Verification items for the finished model (mm, model axes). A direction names the side the tool comes from. Coordinates: 2 decimals unless noted, no trailing zeros. Write each loop counter-clockwise with the first axis right and the second up, starting at its lowest first coordinate (ties: lowest second). Pieces come first, ordered by that corner, then holes. Notation, with made-up numbers: (69.25, 61) -> (74.25, 61) arc R32 cw to (74.25, 95) -> close; hole circle Ø6 at (-19, 20). An arc over 180 degrees is marked (long way). Answer in a Markdown table with one row per item.
```python
from build123d import *

# Parameters (mm, degrees)
SKETCH038_W      = 110
SKETCH038_H      = 32.6
PAD020_DEPTH     = 5
SKETCH039_R      = 1.6
POCKET018_DEPTH  = 5
SKETCH040_W      = 10
SKETCH040_H      = 21.4
SKETCH040_H_2    = 10
PAD021_DEPTH     = 35
MIRROREDSKETCH_R = 1.6
PAD022_DEPTH     = 5
POCKET019_DEPTH  = 110
FILLET012_R      = 2.5


with BuildPart() as part:
    # Sketch038 → Pad020 (new body)
    with BuildSketch(Plane.XY):
        Rectangle(SKETCH038_W, SKETCH038_H)
    extrude(amount=-PAD020_DEPTH)

    # Sketch039 (on Face6 of Pad020) → Pocket018 (cut)
    with BuildSketch(Plane(origin=(0, 0, -5), x_dir=(1, 0, 0), z_dir=(0, 0, -1))):
        with Locations((-37.5, 11.5)):
            Circle(SKETCH039_R)
        with Locations((-37.5, -11.5)):
            Circle(SKETCH039_R)
        with Locations((37.5, -11.5)):
            Circle(SKETCH039_R)
        with Locations((37.5, 11.5)):
            Circle(SKETCH039_R)
    extrude(amount=-POCKET018_DEPTH, mode=Mode.SUBTRACT)

    # Sketch040 (on Face4 of Pocket018) → Pad021 (join)
    with BuildSketch(Plane.XY):
        with Locations((-50, 17)):
            Rectangle(SKETCH040_W, SKETCH040_H)
        with Locations((50, 17)):
            Rectangle(SKETCH040_W, SKETCH040_H)
        with Locations((50, -11.3)):
            Rectangle(SKETCH040_W, SKETCH040_H_2)
        with Locations((-50, -11.3)):
            Rectangle(SKETCH040_W, SKETCH040_H_2)
    extrude(amount=-PAD021_DEPTH)

    # MirroredSketch (on Face35 of Pad021) → Pad022 (join)
    with BuildSketch(Plane(origin=(0, 0, -35), x_dir=(1, 0, 0), z_dir=(0, 0, -1))):
        with BuildLine():
            Line((-45, -27.7), (-45, -6.3))
            Line((-45, -6.3), (-55, -6.3))
            Line((-55, -6.3), (-55, -27.7))
            Line((-55, -27.7), (-55, -30.7))
            ThreePointArc((-55, -30.7), (-50, -35.7), (-45, -30.7))
            Line((-45, -27.7), (-45, -30.7))
        make_face()
        with Locations((-50, -30.7)):
            Circle(MIRROREDSKETCH_R, mode=Mode.SUBTRACT)
        with BuildLine():
            Line((55, -27.7), (55, -6.3))
            Line((55, -6.3), (45, -6.3))
            Line((45, -6.3), (45, -27.7))
            Line((45, -27.7), (45, -30.7))
            ThreePointArc((45, -30.7), (49.999989, -35.7), (55, -30.700021))
            Line((55, -27.7), (55, -30.700021))
        make_face()
        with Locations((50, -30.7)):
            Circle(MIRROREDSKETCH_R, mode=Mode.SUBTRACT)
        with BuildLine():
            Line((45, 6.3), (55, 6.3))
            Line((55, 6.3), (55, 16.3))
            Line((55, 16.3), (55, 19.3))
            ThreePointArc((55, 19.3), (50, 24.3), (45, 19.3))
            Line((45, 16.3), (45, 19.3))
            Line((45, 16.3), (45, 6.3))
        make_face()
        with Locations((50, 19.3)):
            Circle(MIRROREDSKETCH_R, mode=Mode.SUBTRACT)
        with BuildLine():
            Line((-55, 6.3), (-45, 6.3))
            Line((-45, 6.3), (-45, 16.3))
            Line((-45, 16.3), (-45, 19.3))
            ThreePointArc((-45, 19.3), (-50, 24.3), (-55, 19.3))
            Line((-55, 16.3), (-55, 19.3))
            Line((-55, 16.3), (-55, 6.3))
        make_face()
        with Locations((-50, 19.3)):
            Circle(MIRROREDSKETCH_R, mode=Mode.SUBTRACT)
    extrude(amount=PAD022_DEPTH)

    # Sketch041 (on Face44 of Pad022) → Pocket019 (cut)
    with BuildSketch(Plane.YZ.offset(55)):
        Polygon((16.3, 0), (27.7, -35), (27.7, 0), align=None)
        Polygon((17.7, -40), (6.3, -5), (6.3, -40), align=None)
    extrude(amount=-POCKET019_DEPTH, mode=Mode.SUBTRACT)

    # Fillet012
    fillet012_edges = [part.edges().sort_by_distance(p)[0] for p in [
        (-50, 6.3, -5),
        (50, 6.3, -5),
    ]]
    fillet(fillet012_edges, radius=FILLET012_R)


solid = part.part
```
1. Sectioned sample at A-A, the plane x = -50. Record the cut outline in (y, z), and give its area (3 significant figures).
Findings below:
| item | result |
|---|---|
| outline | (-24.3, -40) -> (-20.9, -40) -> (-20.9, -35) -> (-24.3, -35) -> close; (-17.7, -40) -> (-6.3, -40) -> (-6.3, -5) -> (4.49, -5) arc R2.5 cw to (6.86, -6.73) -> (17.7, -40) -> (29.1, -40) -> (29.1, -35) -> (27.7, -35) -> (16.3, 0) -> (-16.3, 0) -> (-16.3, -35) -> (-17.7, -35) -> close; (32.3, -40) -> (35.7, -40) -> (35.7, -35) -> (32.3, -35) -> close |
| area | 969 mm² |
2. Sectioned sample at C-C, the plane y = 20.5. Record the cut outline in (x, z).
Findings below:
| item | result |
|---|---|
| outline | (-55, -40) -> (-45, -40) -> (-45, -12.89) -> (-55, -12.89) -> close; (45, -40) -> (55, -40) -> (55, -12.89) -> (45, -12.89) -> close |
3. Sectioned sample at B-B, the plane z = -20. Record the cut outline in (x, y), and give its area (3 significant figures).
Findings below:
| item | result |
|---|---|
| outline | (-55, -16.3) -> (-45, -16.3) -> (-45, -6.3) -> (-55, -6.3) -> close; (-55, 11.19) -> (-45, 11.19) -> (-45, 22.81) -> (-55, 22.81) -> close; (45, -16.3) -> (55, -16.3) -> (55, -6.3) -> (45, -6.3) -> close; (45, 11.19) -> (55, 11.19) -> (55, 22.81) -> (45, 22.81) -> close |
| area | 433 mm² |
4. Go/stop test with flat-tipped pins: pin 1 (1.9 mm diameter, centred on x = 50, y = -19.3, fed in from +Z); pin 2 (5 mm diameter, centred on x = -47.5, z = -31, fed in from +Y); pin 3 (2.5 mm diameter, centred on x = -49.5, y = 33.5, fed in from +Z); pin 4 (2 mm diameter, centred on x = 34.5, y = 17, fed in from -Z). Record where each tip stops, or that it passes through.
Findings below:
| item | result |
|---|---|
| pin 1 | passes through |
| pin 2 | stops at y = 27.21 |
| pin 3 | stops at z = -35 |
| pin 4 | stops at z = -5 |
5. Release check for a two-part mould opening along Y. For faces 1 (the face through (55, 11, -15)), 2 (the face through (-37.85, 13.06, -2.54)), 3 (the face through (-4, -16.3, -4)), 4 (the face through (49.9, 35.7, -37.5)) record: released by +Y, released by -Y, zero draft, split by the parting line, or undercut.
Findings below:
| item | result |
|---|---|
| face 1 | zero draft |
| face 2 | undercut |
| face 3 | released by -Y |
| face 4 | released by +Y |
6. Access from +Z, -Z, +X, -X, +Y, -Y to the whole of each face (thin tool, end or side, straight path). Record for faces 5 (the face through (-38.68, -12.58, -2.54)), 6 (the face through (50.07, 5.936, -5.464)), 7 (the face through (-45, -11, -22)), 8 (the face through (-50, 33, -35)), 9 (the face through (-49.9, -24.3, -37.5)).
Findings below:
| item | result |
|---|---|
| face 5 | +Z, -Z |
| face 6 | -Z, +X, -X |
| face 7 | -Z, +Y, -Y |
| face 8 | +Z, +X, -X, +Y |
| face 9 | +Z, -Z, -Y |
7. Material ranges on probe 1 along X at (y, z) = (30.7, -38.5); probe 2 along Y at (x, z) = (-37.5, -2.45); probe 3 along Y at (x, z) = (50, -37.25), recorded low to high. Write a range as from..to.
Findings below:
| item | result |
|---|---|
| probe 1 | x = -55..-51.6, -48.4..-45, 45..48.4, 51.6..55 |
| probe 2 | y = -16.3..-13.1, -9.9..9.9, 13.1..16.3 |
| probe 3 | y = -24.3..-20.9, -17.7..-6.3, 16.8..29.1, 32.3..35.7 |
8. Sectioned sample at D-D, the plane x = 37.5. Record the cut outline in (y, z).
Findings below:
| item | result |
|---|---|
| outline | (-16.3, -5) -> (-13.1, -5) -> (-13.1, 0) -> (-16.3, 0) -> close; (-9.9, -5) -> (9.9, -5) -> (9.9, 0) -> (-9.9, 0) -> close; (13.1, -5) -> (16.3, -5) -> (16.3, 0) -> (13.1, 0) -> close |
